The drawing under review shows one solid part. Ordinate dimensions are in mm from its lowest x, y, z. Coordinates: 2 decimals unless noted, no trailing zeros. Loops run counter-clockwise (first coordinate to the right, second up) from the corner with the lowest first, then second, coordinate; pieces in that order, holes last. Notation, with made-up numbers: (72.25, 49.5) - (88.25, 49.5) arc R26 ccw to (88.25, 67.5) - close; hole circle Ø1 at (-4.75, -28.5). An arc over 180 degrees is marked (long way). Use one line per item in the form item = value. Start each with the question number.
1. To check wall thickness, follow probe 1 along Y at (x, z) = (0.9, 0.7); probe 2 along Y at (x, z) = (2.1, 3.65). State the ranges of each line that lie inside material, in increasing order.
2. For pin 1 Ø2 at (x, z) = (0.5, 0.5) entering from +Y, flat-tipped, find the tip position at first contact; note if it passes through.
3. Add section B-B on z = 2.5. Give the boundary of the cut face in (x, y), and give its area (3 significant figures).
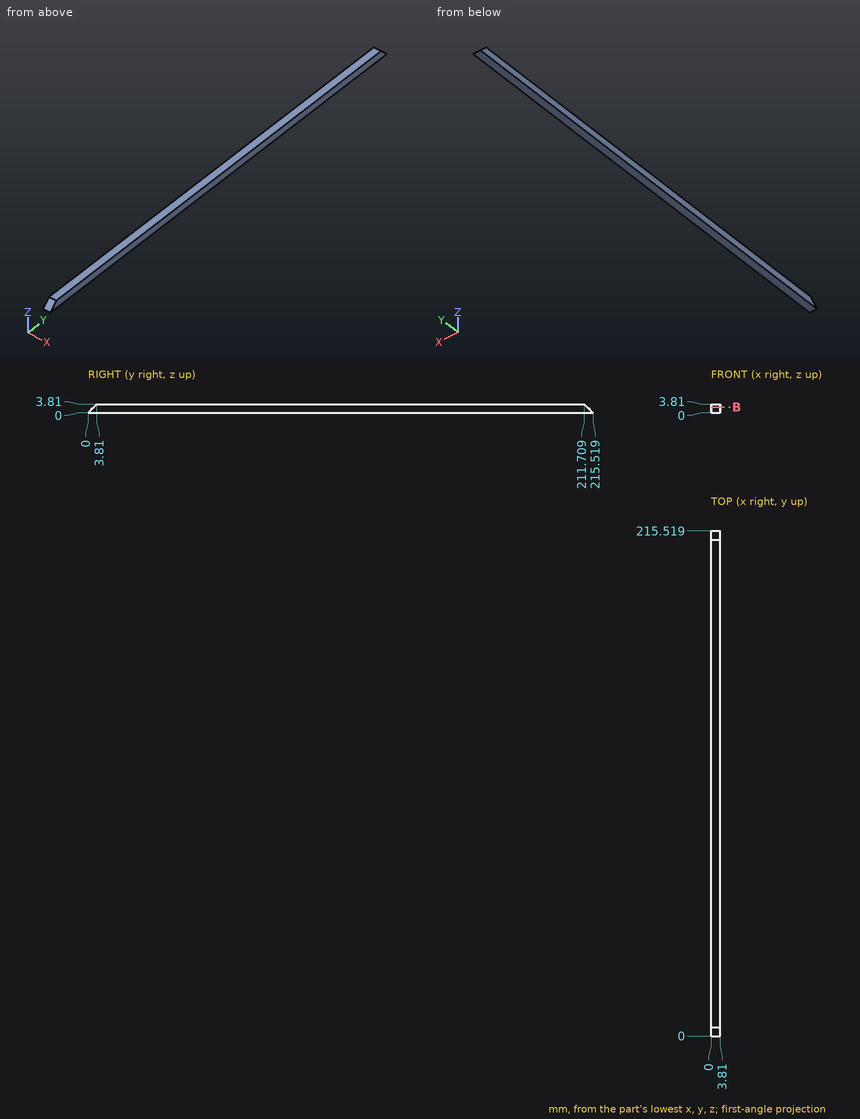
Conclusion:
q1.probe_1 = 0.7 to 214.82
q1.probe_2 = 3.65 to 211.87
q2.pin_1 = 215.52
q3.outline = (0, 2.5) - (3.81, 2.5) - (3.81, 213.02) - (0, 213.02) - close
q3.area = 802 mm^2
